from build123d import *

# Parameters (mm, degrees)
ESQUISSE3_W                  = 7.5
ESQUISSE3_H                  = 5.8
ENL_V_MAT_EXTRU_1_DEPTH      = 8
CONG_1_R                     = 0.5
ENL_V_MAT_EXTRU_2_DEPTH      = 89.156310052
ENL_V_MAT_EXTRU_2_DEPTH_BACK = 89.156310052
ESQUISSE4_R                  = 0.75
ESQUISSE5_W                  = 0.75
ESQUISSE5_H                  = 3.75
ESQUISSE5_W_2                = 2.511980861
ESQUISSE5_H_2                = 0.75
BOSS_EXTRU_1_DEPTH           = 0.2
CONG_2_R                     = 0.2
CONG_2_OF_SYM_TRIE1_R        = 0.2
ENL_V_MAT_EXTRU_3_DEPTH      = 89.360030571


with BuildPart() as part:
    # Esquisse2 → Révolution1 (revolve)
    with BuildSketch(Plane.XY, mode=Mode.PRIVATE) as r_volution1_sk:
        with BuildLine():
            Line((4.014003451, 30.213287326), (4.735996549, 20.586712674))
            ThreePointArc((4.735996549, 20.586712674), (4.746497911, 20.399868856), (4.75, 20.212762933))
            Line((4.75, 20.212762933), (4.75, 0))
            Line((4.75, 0), (1, 0))
            Line((1, 0), (1, 83.9))
            Line((1, 83.9), (0, 83.9))
            Line((0, 83.9), (0, 87.9))
            ThreePointArc((0, 87.9), (2.828427125, 86.728427125), (4, 83.9))
            Line((4, 83.9), (4, 78.6))
            Line((4, 78.6), (3.75, 78.6))
            Line((3.75, 78.6), (3.75, 78.1))
            Line((3.75, 78.1), (4, 78.1))
            Line((4, 78.1), (4, 77.1))
            Line((4, 77.1), (3.75, 77.1))
            Line((3.75, 77.1), (3.75, 76.6))
            Line((3.75, 76.6), (4, 76.6))
            Line((4, 76.6), (4, 30.587237067))
            ThreePointArc((4, 30.587237067), (4.003502089, 30.400131144), (4.014003451, 30.213287326))
        make_face()
    revolve(r_volution1_sk.sketch.rotate(Axis((0, 0, 0), (0, 1, 0)), 90), axis=Axis((0, 0, 0), (0, 1, 0)))

    # Esquisse3 → Enlèv. mat.-Extru.1 (cut)
    with BuildSketch(Plane.XZ):
        with Locations((1, 0)):
            Rectangle(ESQUISSE3_W, ESQUISSE3_H)
    extrude(amount=-ENL_V_MAT_EXTRU_1_DEPTH, mode=Mode.SUBTRACT)

    # Congé1
    cong_1_edges = [part.edges().sort_by_distance(p)[0] for p in [
        (-4.262481672, 0, 2.096127382),
    ]]
    fillet(cong_1_edges, radius=CONG_1_R)

    # Esquisse4 → Enlèv. mat.-Extru.2 (cut, two sides: drawn at the far end of the back side and taken through both)
    with BuildSketch(Plane.XY.offset(-ENL_V_MAT_EXTRU_2_DEPTH_BACK)):
        with Locations(Location((0, 5, 0), (0, 0, 90))):
            Circle(ESQUISSE4_R)
        with BuildLine():
            Line((1.161980861, 0), (3.761980861, 0))
            Line((3.761980861, 0), (3.761980861, 2.6))
            ThreePointArc((3.761980861, 2.6), (3.000458492, 0.761522369), (1.161980861, 0))
        make_face()
        Polygon((3.761980861, 8), (4.75, 10), (4.75, 8), align=None)
    extrude(amount=ENL_V_MAT_EXTRU_2_DEPTH + ENL_V_MAT_EXTRU_2_DEPTH_BACK, mode=Mode.SUBTRACT)

    # Esquisse5 → Boss.-Extru.1 (add)
    with BuildSketch(Plane.XY.offset(-2.9)):
        with Locations((0, 1.875)):
            Rectangle(ESQUISSE5_W, ESQUISSE5_H)
        Polygon((0.618718434, 3.850951481), (1.149048519, 4.381281566), (4.027145904, 1.503184182), (3.496815818, 0.972854096), align=None)
        with Locations((2.50599043, 5)):
            Rectangle(ESQUISSE5_W_2, ESQUISSE5_H_2)
    boss_extru_1 = extrude(amount=BOSS_EXTRU_1_DEPTH)

    # Congé2
    cong_2_edges = [part.edges().sort_by_distance(p)[0] for p in [
        (2.505990431, 5.375, -2.7),
        (2.505990431, 4.625, -2.7),
        (2.588097212, 2.942232874, -2.7),
        (2.057767126, 2.411902788, -2.7),
        (-0.375, 1.875, -2.7),
        (0.375, 1.875, -2.7),
    ]]
    fillet(cong_2_edges, radius=CONG_2_R - 0.0001)  # a hair under: the kernel refuses the full size

    # Symétrie1: Boss.-Extru.1 across plane
    add(boss_extru_1.mirror(Plane.XY))

    # Congé2 of Symétrie1
    cong_2_of_sym_trie1_edges = [part.edges().sort_by_distance(p)[0] for p in [
        (2.505990431, 5.375, 2.7),
        (2.505990431, 4.625, 2.7),
        (2.588097212, 2.942232874, 2.7),
        (2.057767126, 2.411902788, 2.7),
        (-0.375, 1.875, 2.7),
        (0.375, 1.875, 2.7),
    ]]
    fillet(cong_2_of_sym_trie1_edges, radius=CONG_2_OF_SYM_TRIE1_R - 0.0001)  # a hair under: the kernel refuses the full size

    # Esquisse6 → Enlèv. mat.-Extru.3 (cut, through all)
    with BuildSketch(Plane.XY.offset(2.9)):
        with BuildLine():
            Line((4.027145904, 1.503184182), (3.658059706, 1.87227038))
            ThreePointArc((3.658059706, 1.87227038), (3.516870908, 1.49795968), (3.319930166, 1.149739748))
            Line((3.319930166, 1.149739748), (3.496815818, 0.972854096))
            Line((3.496815818, 0.972854096), (4.027145904, 1.503184182))
        make_face()
    extrude(amount=-ENL_V_MAT_EXTRU_3_DEPTH, mode=Mode.SUBTRACT)


solid = part.part
Could you check a few things on this model? Use its own coordinates, in mm. A direction names the side the tool comes from. Give positions to 0.01 mm unless a question says otherwise; leave off trailing zeros. Order: outer loops, then holes, each group sorted by start corner. A loop starts at its lowest first (then second) coordinate and runs counter-clockwise, first axis right, second up. Notation, with made-up numbers: (71.25, 80.5) - (128.25, 80.5) arc R19 cw to (128.25, 115.5) - close; hole circle Ø4 at (18, 59). An arc over 180 degrees is marked (long way). One line per item, written item: value. Start each with the question number.
1. If I drill on probe 1 along X at (y, z) = (65, 0); probe 2 along Z at (x, y) = (2, 4); probe 3 along X at (y, z) = (5, 3.3), over which ranges is the centre line in solid material (lowest first)?
2. Thinking about a two-plate mould opening in Y: for faces 1 (the face through (2, 3, 2.7)), 2 (the face through (1.99, 2.56, -2.76)), 3 (the face through (2.42, 3.03, -2.76)), which applies, +Y half, -Y half, draft (parallel to the pull), parting line (faces both ways), or undercut?
3. For P1, Ø5, axis at y = 61, z = 1.5, coming from the +X side; P2, Ø1.5, axis at x = -1, y = 17.5, coming from the +Z side; P3, Ø5, axis at x = 2, z = -3.5, coming from the +Y side; P4, Ø4, axis at x = -0.5, z = -1.5, coming from the -Y side, each with a flat end and sliding along its axis, tell me the tip position at first contact or that it passes through.
4. For faces 4 (the face through (3.905, 77.593, 0.867)), 5 (the face through (1.99, 2.56, 2.76)), 6 (the face through (0, 4, 2.9)), which set-ups out of +Z, -Z, +X, -X, +Y, -Y let a thin tool reach every point of the face, with its end or its side?
5. Imagine slicing it at A-A on y = 75. List the corners of the cut face in (x, z) for me, plus the area to 3 significant figures.
Values:
1. probe 1: -4 to -1, 1 to 4
1. probe 2: -4.31 to -2.9, 2.9 to 4.31
1. probe 3: -3.42 to -0.75, 0.75 to 3.42
2. face 1: draft
2. face 2: -Y half
2. face 3: undercut
3. P1: x = 4
3. P2: z = 4.74
3. P3: y = 87.6
3. P4: y = 0
4. face 4: +Y
4. face 5: -Y
4. face 6: none
5. outline: circle Ø8 at (0, 0); hole circle Ø2 at (0, 0)
5. area: 47.1 mm²
